Input: part model. Units: mm. Frame: model coordinates. Face numbers are marked on the shaded views. A direction names the side the tool comes from. Coordinates: 2 decimals unless noted, no trailing zeros. Loops run counter-clockwise (first coordinate to the right, second up) from the corner with the lowest first, then second, coordinate; pieces in that order, holes last. Notation, with made-up numbers: (-25.75, 75.5) -> (32.25, 75.5) arc R13 cw to (32.25, 100.5) -> close; hole circle Ø6 at (22, 60.25). An arc over 180 degrees is marked (long way). Answer as a JSON object with one key per item and string values.
from build123d import *
from OCP.BRepFilletAPI import BRepFilletAPI_MakeChamfer

# Parameters (mm, degrees)
SKETCH1_W               = 3.5
SKETCH1_H               = 12
SKETCH2_R               = 2.2
CUT_EXTRUDE1_DEPTH      = 23
SKETCH3_R               = 2
CUT_EXTRUDE2_DEPTH      = 9
CUT_EXTRUDE3_DEPTH      = 36.864327681
CUT_EXTRUDE4_DEPTH      = 36.864327798
CUT_EXTRUDE5_DEPTH      = 0.3
CUT_EXTRUDE5_DEPTH_BACK = 0.3
CUT_EXTRUDE8_DEPTH      = 0.3
CUT_EXTRUDE8_DEPTH_BACK = 0.3
CUT_EXTRUDE7_START      = 5.3
SKETCH15_R              = 3.5
SKETCH15_R_2            = 3
CUT_EXTRUDE7_DEPTH      = 5.3
CHAMFER1_SIZE           = 0.4
CHAMFER1_SIZE2          = 0.407141204


# Read off the part's stored shape, not the designer's step: CSK for M3 Oval Head Machine Screw1
with BuildPart() as part:
    # Sketch1 → Revolve1 (revolve)
    with BuildSketch(Plane.XY):
        Polygon((0, 12), (3.5, 12), (3.1, 35), (0, 35), align=None)
        with Locations((1.75, 6)):
            Rectangle(SKETCH1_W, SKETCH1_H)
    revolve(axis=Axis((0, 0, 0), (0, 1, 0)))

    # Sketch2 → Cut-Extrude1 (cut)
    with BuildSketch(Plane(origin=(0, 35, 0), x_dir=(1, 0, 0), z_dir=(0, 1, 0))):
        with Locations(Location((0, 0, 0), (0, 0, 270))):
            Circle(SKETCH2_R)
    extrude(amount=-CUT_EXTRUDE1_DEPTH, mode=Mode.SUBTRACT)

    # Sketch3 → Cut-Extrude2 (cut)
    with BuildSketch(Plane.XZ):
        with Locations(Location((0, -0.502631205, 0), (0, 0, 270))):
            Circle(SKETCH3_R)
    extrude(amount=-CUT_EXTRUDE2_DEPTH, mode=Mode.SUBTRACT)

    # Sketch5 → Cut-Extrude3 (cut, through all)
    with BuildSketch(Plane.ZY.offset(3.5)):
        Polygon((0.3, 12), (-0.3, 12), (-0.005, 35), (0.005, 35), align=None)
    extrude(amount=-CUT_EXTRUDE3_DEPTH, mode=Mode.SUBTRACT)

    # Sketch9 → Cut-Extrude4 (cut, through all)
    with BuildSketch(Plane.XY.offset(3.5)):
        Polygon((0.305, 12), (-0.295, 12), (0, 35), (0.01, 35), align=None)
    extrude(amount=-CUT_EXTRUDE4_DEPTH, mode=Mode.SUBTRACT)

    # Sketch11 → Cut-Extrude5 (cut, two sides: drawn at the far end of the back side and taken through both)
    with BuildSketch(Plane.XY.offset(-CUT_EXTRUDE5_DEPTH_BACK)):
        Polygon((-0.249466739, 12.5), (-3.597980128, 12.5), (-3.500702869, 6.5), align=None)
        Polygon((3.597980128, 12.5), (3.500702869, 6.5), (0.249466739, 12.5), align=None)
    extrude(amount=CUT_EXTRUDE5_DEPTH + CUT_EXTRUDE5_DEPTH_BACK, mode=Mode.SUBTRACT)

    # Sketch22 → Cut-Extrude8 (cut, two sides: drawn at the far end of the back side and taken through both)
    with BuildSketch(Plane(origin=(0, 0, 0), x_dir=(0, 0, -1), z_dir=(1, 0, 0)).offset(-CUT_EXTRUDE8_DEPTH_BACK)):
        Polygon((3.5, 7.3), (2.2, 12), (3.618391535, 12), align=None)
        Polygon((-2.2, 12), (-3.5, 12), (-3.5, 7.3), align=None)
    extrude(amount=CUT_EXTRUDE8_DEPTH + CUT_EXTRUDE8_DEPTH_BACK, mode=Mode.SUBTRACT)

    # Sketch15 → Cut-Extrude7 (cut)
    with BuildSketch(Plane(origin=(0, 28, 0), x_dir=(1, 0, 0), z_dir=(0, 1, 0)).offset(CUT_EXTRUDE7_START)):
        Circle(SKETCH15_R)
        Circle(SKETCH15_R_2, mode=Mode.SUBTRACT)
    extrude(amount=-CUT_EXTRUDE7_DEPTH, mode=Mode.SUBTRACT)

    # CSK for M3 Oval Head Machine Screw1 outl → CSK for M3 Oval Head Machine Screw1 (revolve, cut)
    with BuildSketch(Plane.XZ.offset(-3.6)):
        Polygon((0, 0.819848747), (1.5, 0.819848747), (1.5, 2.75), (2.250138013, 3.500138013), (0, 3.500138013), align=None)
    revolve(axis=Axis((0, 3.6, 0), (0, 0, 1)), mode=Mode.SUBTRACT)

    # Chamfer1: one chamfer whose edges measure the first distance from different faces: ONE call of the kernel's chamfer builder (chamfer() names one face for all edges)
    chamfer1_edges_1 = [part.edges().sort_by_distance(p)[0] for p in [
        (-2.190262541, 35, 2.193798076),
    ]]
    chamfer1_side_1 = [part.faces().sort_by_distance(p)[0] for p in [
        (-2.200706991, 34.15, 2.204259386),
    ]]
    chamfer1_edges_2 = [part.edges().sort_by_distance(p)[0] for p in [
        (2.193798081, 35, 2.190262537),
    ]]
    chamfer1_side_2 = [part.faces().sort_by_distance(p)[0] for p in [
        (2.20425939, 34.15, 2.200706986),
    ]]
    chamfer1_edges_3 = [part.edges().sort_by_distance(p)[0] for p in [
        (2.193798081, 35, -2.190262537),
    ]]
    chamfer1_side_3 = [part.faces().sort_by_distance(p)[0] for p in [
        (2.20425939, 34.15, -2.200706986),
    ]]
    chamfer1_edges_4 = [part.edges().sort_by_distance(p)[0] for p in [
        (-2.190262541, 35, -2.193798076),
    ]]
    chamfer1_side_4 = [part.faces().sort_by_distance(p)[0] for p in [
        (-2.200706991, 34.15, -2.204259386),
    ]]
    chamfer1_edges_5 = [part.edges().sort_by_distance(p)[0] for p in [
        (-1.553866146, 35, 1.557401682),
        (1.557401691, 35, 1.553866137),
        (1.557401691, 35, -1.553866137),
        (-1.553866146, 35, -1.557401682),
        (0, 0, 1.497368795),
    ]]
    chamfer1 = BRepFilletAPI_MakeChamfer(part.part.solid().wrapped)
    for e in chamfer1_edges_1:
        chamfer1.Add(CHAMFER1_SIZE, CHAMFER1_SIZE2, e.wrapped, chamfer1_side_1[0].wrapped)  # the first distance lies on this face
    for e in chamfer1_edges_2:
        chamfer1.Add(CHAMFER1_SIZE, CHAMFER1_SIZE2, e.wrapped, chamfer1_side_2[0].wrapped)  # the first distance lies on this face
    for e in chamfer1_edges_3:
        chamfer1.Add(CHAMFER1_SIZE, CHAMFER1_SIZE2, e.wrapped, chamfer1_side_3[0].wrapped)  # the first distance lies on this face
    for e in chamfer1_edges_4:
        chamfer1.Add(CHAMFER1_SIZE, CHAMFER1_SIZE2, e.wrapped, chamfer1_side_4[0].wrapped)  # the first distance lies on this face
    for e in chamfer1_edges_5:
        chamfer1.Add(CHAMFER1_SIZE, e.wrapped)
    add(Compound.cast(chamfer1.Shape()), mode=Mode.REPLACE)


solid = part.part
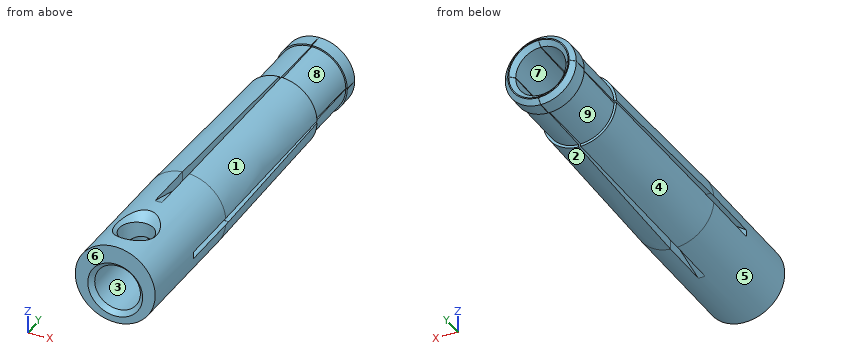
1. Line query: line 1 along Y through (x, z) = (0, 1.9); line 2 along Y through (x, z) = (0, 1.8); line 3 along Z through (x, y) = (0.75, 25.5). Output: solid intervals per line, ascending.
Reply:
{"line 1": "y = 0 to 2.1, 5.1 to 12", "line 2": "y = 0.1 to 2.1, 5.1 to 12", "line 3": "z = -3.18 to -2.07, 2.07 to 3.18"}
2. Mould query, pull axis Y, two halves, no side actions, for the marked faces 6, 7, 8 and 9. Classes: pulls with the +Y half, pulls with the -Y half, needs draft (parallel to the pull), parting line crosses it, or undercut.
Reply:
{"face 6": "pulls with the -Y half", "face 7": "needs draft", "face 8": "undercut", "face 9": "undercut"}
3. Access query for the marked faces 1, 2, 3, 4 and 5. Directions: +Z, -Z, +X, -X, +Y, -Y. A direction counts if a zero-diameter tool reaches every point of the face in a straight line with its end or side. Return the directions, or none.
Reply:
{"face 1": "+Z, +X, +Y", "face 2": "-Z, +X, +Y", "face 3": "-Y", "face 4": "-Z, -X, +Y", "face 5": "+Y, -Y"}
4. Section query C-C (y = 15). Return loops of the section in (x, z) (1 decimal).
Reply:
{"outline": "(-3.4, -0.3) arc R3.4 ccw to (-0.3, -3.4) -> (-0.3, -2.2) arc R2.2 cw to (-2.2, -0.3) -> close; (-3.4, 0.3) -> (-2.2, 0.3) arc R2.2 cw to (-0.3, 2.2) -> (-0.3, 3.4) arc R3.4 ccw to start; (0.3, -3.4) arc R3.4 ccw to (3.4, -0.3) -> (2.2, -0.3) arc R2.2 cw to (0.3, -2.2) -> close; (0.3, 2.2) arc R2.2 cw to (2.2, 0.3) -> (3.4, 0.3) arc R3.4 ccw to (0.3, 3.4) -> close"}
5. Pin query (flat end, axial travel): P1, Ø1, axis at y = 10, z = -2.5, coming from the +X side; P2, Ø2.5, axis at x = 0, z = -0.5, coming from the -Y side; P3, Ø1, axis at y = 15, z = -0.5, coming from the -X side. Return the tip coordinate at first contact, or that it passes through.
Reply:
{"P1": "stops at x = 2.87", "P2": "stops at y = 9", "P3": "stops at x = -3.45"}
6. Section query B-B (y = 3.6). Return loops of the section in (x, z).
Reply:
{"outline": "(-1.77, 3.02) arc R3.5 ccw (long way) to (1.77, 3.02) -> (1.5, 2.75) -> (1.5, 0.82) arc R2 cw (long way) to (-1.5, 0.82) -> (-1.5, 2.75) -> close"}
7. Section query A-A (y = 29.5). Return loops of the section in (x, z), plus the area to 3 significant figures.
Reply:
{"outline": "(-3, -0.08) arc R3 ccw to (-0.07, -3) -> (-0.07, -2.2) arc R2.2 cw to (-2.2, -0.08) -> close; (-3, 0.08) -> (-2.2, 0.08) arc R2.2 cw to (-0.07, 2.2) -> (-0.07, 3) arc R3 ccw to start; (0.08, -3) arc R3 ccw to (3, -0.08) -> (2.2, -0.08) arc R2.2 cw to (0.08, -2.2) -> close; (0.08, 2.2) arc R2.2 cw to (2.2, 0.08) -> (3, 0.08) arc R3 ccw to (0.08, 3) -> close", "area": "12.6 mm2"}
